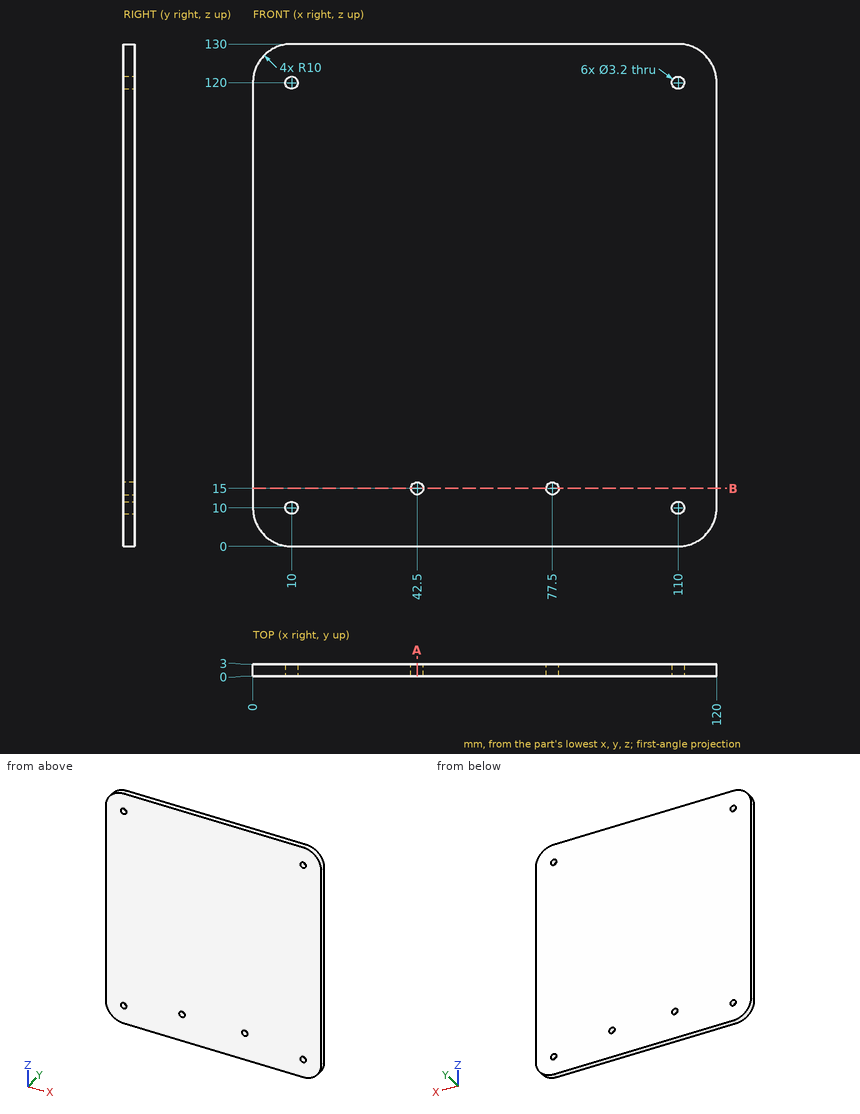
Source: three-view drawing plus pictorial views. Frame: mm from the lowest corner of the part. Round coordinates to 2 decimals unless told otherwise and drop trailing zeros. Order: outer loops, then holes, each group sorted by start corner. A loop starts at its lowest first (then second) coordinate and runs counter-clockwise, first axis right, second up. Notation, with made-up numbers: (-20, 89.5) -> (29, 89.5) arc R24 cw to (29, 123.5) -> close; hole circle Ø1 at (-32.5, -17.5). An arc over 180 degrees is marked (long way). Use CSV: the item, a comma, the result in double quotes. Start each with the question number.
1) Section A-A (x = 42.5). Return the cut outline in (y, z), and give its area (3 significant figures).
2) Section B-B (z = 15). Return the cut outline in (x, y).
3) First-contact query: pin 1 Ø3 at (x, z) = (42.5, 15) entering from -Y. Flat tip, straight axial feed; report the tip coordinate or a pass-through.
4) Material intervals for line 1 along Z through (x, y) = (110, 2.1); line 2 along X through (y, z) = (1.25, 15); line 3 along X through (y, z) = (0.6, 10), sorted ascending. Write a range as from..to.
Returned:
1,outline,"(0, 0) -> (3, 0) -> (3, 13.4) -> (0, 13.4) -> close; (0, 16.6) -> (3, 16.6) -> (3, 130) -> (0, 130) -> close"
1,area,"380 mm²"
2,outline,"(0, 0) -> (40.9, 0) -> (40.9, 3) -> (0, 3) -> close; (44.1, 0) -> (75.9, 0) -> (75.9, 3) -> (44.1, 3) -> close; (79.1, 0) -> (120, 0) -> (120, 3) -> (79.1, 3) -> close"
3,pin 1,"passes through"
4,line 1,"z = 0..8.4, 11.6..118.4, 121.6..130"
4,line 2,"x = 0..40.9, 44.1..75.9, 79.1..120"
4,line 3,"x = 0..8.4, 11.6..108.4, 111.6..120"
